The drawing under review shows one solid part. Ordinate dimensions are in mm from its lowest x, y, z. A direction names the side the tool comes from. Coordinates: 2 decimals unless noted, no trailing zeros. Order: outer loops, then holes, each group sorted by start corner. A loop starts at its lowest first (then second) coordinate and runs counter-clockwise, first axis right, second up. Notation, with made-up numbers: (34, 37) - (82, 37) arc R19 ccw to (82, 46) - close; hole circle Ø9 at (-8, 28). An arc over 180 degrees is marked (long way). Answer in a Markdown table with one row per item.
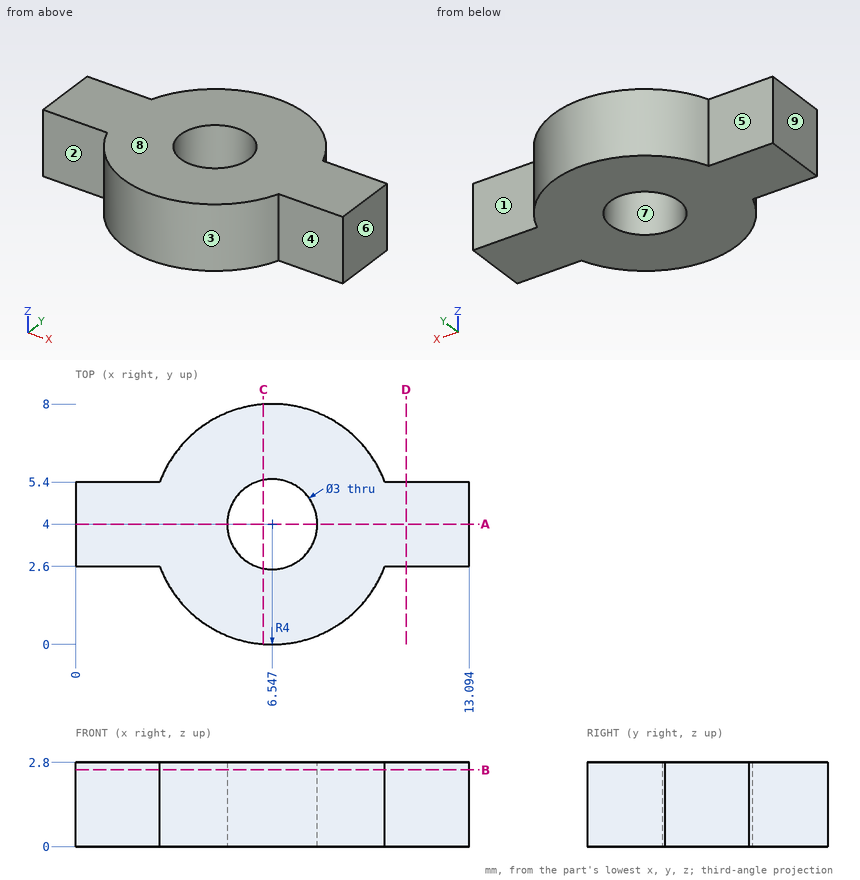
Item 1: Tool access review of the marked faces 1, 2, 3, 4 and 5: name each direction out of +Z, -Z, +X, -X, +Y, -Y from which nothing blocks a thin tool from reaching the whole face with its end or side.
Check values:
| item | result |
|---|---|
| face 1 | +Z, -Z, +X, +Y |
| face 2 | +Z, -Z, -X, -Y |
| face 3 | +Z, -Z, -Y |
| face 4 | +Z, -Z, +X, -Y |
| face 5 | +Z, -Z, -X, +Y |
Item 2: We need section D-D, the plane x = 11. Write out the cut boundary in (y, z).
Check values:
| item | result |
|---|---|
| outline | (2.6, 0) - (5.4, 0) - (5.4, 2.8) - (2.6, 2.8) - close |
Item 3: We need section B-B, the plane z = 2.55. Write out the cut boundary in (x, y).
Check values:
| item | result |
|---|---|
| outline | (0, 2.6) - (2.8, 2.6) arc R4 ccw to (10.29, 2.6) - (13.09, 2.6) - (13.09, 5.4) - (10.29, 5.4) arc R4 ccw to (2.8, 5.4) - (0, 5.4) - close; hole circle Ø3 at (6.55, 4) |
Item 4: Mouldability with a two-part tool opening along X and no side actions: class the marked faces 6, 7, 8 and 9 as +X half, -X half, draft (parallel to the pull), parting line (faces both ways), or undercut.
Check values:
| item | result |
|---|---|
| face 6 | +X half |
| face 7 | undercut |
| face 8 | draft |
| face 9 | -X half |
Item 5: We need section C-C, the plane x = 6.25. Write out the cut boundary in (y, z).
Check values:
| item | result |
|---|---|
| outline | (0.01, 0) - (2.53, 0) - (2.53, 2.8) - (0.01, 2.8) - close; (5.47, 0) - (7.99, 0) - (7.99, 2.8) - (5.47, 2.8) - close |
Item 6: Clearance check with flat-ended pins moving along their axes: pin 1 Ø0.8 at (x, z) = (1, 1.5) entering from -Y; pin 2 Ø1.4 at (x, z) = (11.5, 2) entering from +Y; pin 3 Ø1.5 at (x, z) = (8.5, 0.5) entering from -Y. State where each tip first meets the part, or that it passes through.
Check values:
| item | result |
|---|---|
| pin 1 | y = 2.6 |
| pin 2 | y = 5.4 |
| pin 3 | y = 0.19 |
Item 7: We need section A-A, the plane y = 4. Write out the cut boundary in (x, z), then the cut area to 3 significant figures.
Check values:
| item | result |
|---|---|
| outline | (0, 0) - (5.05, 0) - (5.05, 2.8) - (0, 2.8) - close; (8.05, 0) - (13.09, 0) - (13.09, 2.8) - (8.05, 2.8) - close |
| area | 28.3 mm^2 |
Item 8: To check wall thickness, follow line 1 (Y direction, x = 10.5, z = 0.55); line 2 (Y direction, x = 7.5, z = 1); line 3 (Y direction, x = 7.75, z = 1.2). State the ranges of each line that lie inside material, in increasing order. Write a range as from..to.
Check values:
| item | result |
|---|---|
| line 1 | 2.6..5.4 |
| line 2 | 0.12..2.84, 5.16..7.88 |
| line 3 | 0.19..3.1, 4.9..7.81 |
